Autodesk Inventor part; units mm, degrees
ref_plane "YZ Plane" through (0, 0, 0) normal (1, 0, 0) x (0, 1, 0)
ref_plane "XZ Plane" through (0, 0, 0) normal (0, 1, 0) x (-1, 0, 0)
ref_plane "XY Plane" through (0, 0, 0) normal (0, 0, 1) x (1, 0, 0)
sketch "Skizze1" plane through (0, 0, 0) normal (0, 0, 1) x (1, 0, 0)
  line L0 (-11, -10) -> (11, -10)
  line L1 (11, -10) -> (11, 10)
  line L2 (11, 10) -> (-11, 10)
  line L3 (-11, 10) -> (-11, -10)
extrude "Extrusion1" add sketch "Skizze1" along normal blind 3
sketch "Skizze2" plane through (0, 0, 0) normal (0, 0, 1) x (1, 0, 0)
  circle A0 centre (0, 0) radius 3.3
extrude "Extrusion2" cut sketch "Skizze2" along normal blind 3.2
sketch "Skizze3" plane through (0, 0, 0) normal (0, 0, 1) x (1, 0, 0)
  circle A0 centre (-9, 0) radius 1.2
extrude "Extrusion3" cut sketch "Skizze3" along normal blind 3.2
sketch "Skizze4" plane through (0, 0, 0) normal (0, 0, 1) x (1, 0, 0)
  circle A0 centre (9, 0) radius 1.2
extrude "Extrusion4" cut sketch "Skizze4" along normal blind 3.2
properties part number "Taststift_Kappe"
Geometry check sheet. Reference: the model listing, model coordinates, mm. Give positions to 0.01 mm unless a question says otherwise; leave off trailing zeros. Loops run counter-clockwise (first coordinate to the right, second up) from the corner with the lowest first, then second, coordinate; pieces in that order, holes last. Notation, with made-up numbers: (60, 88) -> (110, 88) arc R30 ccw to (110, 114) -> close; hole circle Ø11 at (58, 77). An arc over 180 degrees is marked (long way). Answer in a Markdown table with one row per item. Add a question column.
1) Cross-section at B-B on x = -9. Record the boundary of the cut face in (y, z).
2) Draft check along Y on faces 1 (the face through (-3, 2, 0)), 2 (the face through (-10.2, -0.05, 1.48)), 3 (the face through (0, -10, 1)). Enter one of: pulls with the +Y half, pulls with the -Y half, needs draft (parallel to the pull), parting line crosses it, or undercut.
3) Material ranges on probe 1 along X at (y, z) = (0, 0.85); probe 2 along Y at (x, z) = (9, 2.2); probe 3 along X at (y, z) = (1, 0.6), recorded low to high. Write a range as from..to.
4) Cross-section at C-C on y = 1.75. Record the boundary of the cut face in (x, z).
5) Cross-section at A-A on z = 1.85. Record the boundary of the cut face in (x, y), and give its area (3 significant figures).
Outcome:
| question | item | result |
|---|---|---|
| 1 | outline | (-10, 0) -> (-1.2, 0) -> (-1.2, 3) -> (-10, 3) -> close; (1.2, 0) -> (10, 0) -> (10, 3) -> (1.2, 3) -> close |
| 2 | face 1 | needs draft |
| 2 | face 2 | undercut |
| 2 | face 3 | pulls with the -Y half |
| 3 | probe 1 | x = -11..-10.2, -7.8..-3.3, 3.3..7.8, 10.2..11 |
| 3 | probe 2 | y = -10..-1.2, 1.2..10 |
| 3 | probe 3 | x = -11..-9.66, -8.34..-3.14, 3.14..8.34, 9.66..11 |
| 4 | outline | (-11, 0) -> (-2.8, 0) -> (-2.8, 3) -> (-11, 3) -> close; (2.8, 0) -> (11, 0) -> (11, 3) -> (2.8, 3) -> close |
| 5 | outline | (-11, -10) -> (11, -10) -> (11, 10) -> (-11, 10) -> close; hole circle Ø2.4 at (-9, 0); hole circle Ø6.6 at (0, 0); hole circle Ø2.4 at (9, 0) |
| 5 | area | 397 mm^2 |
